Source: three-view drawing plus pictorial views. Frame: mm from the lowest corner of the part. Coordinates: 2 decimals unless noted, no trailing zeros. Write each loop counter-clockwise with the first axis right and the second up, starting at its lowest first coordinate (ties: lowest second). Pieces come first, ordered by that corner, then holes. Notation, with made-up numbers: M 8.5,31 L 32.5,31 A18 ccw 32.5,62 Z; hole C -20.5,69.25 d8. An arc over 180 degrees is marked long. Use CSV: the item, a comma, the result in double quotes.
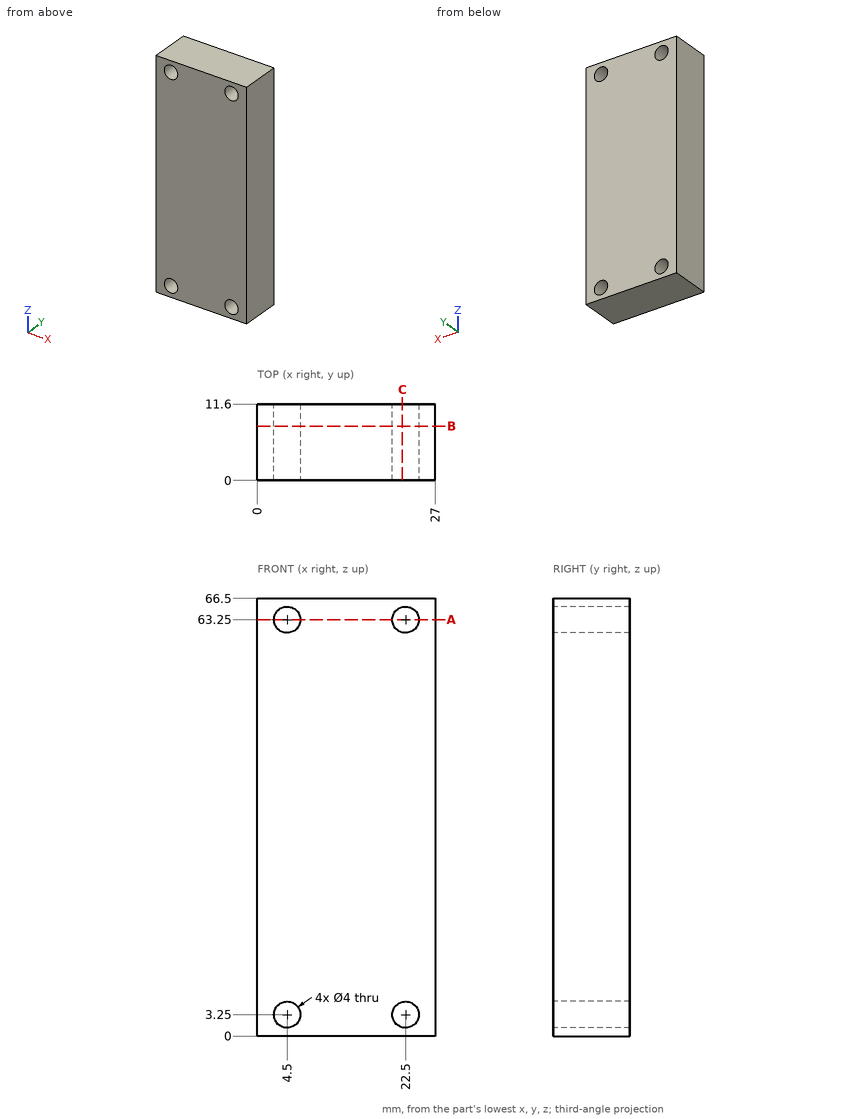
1. Material intervals for line 1 (Z direction, x = 4.5, y = 3.75); line 2 (Z direction, x = 5.25, y = 7.5), sorted ascending. Write a range as [from, to].
Resolved:
line 1,"z = [0, 1.25], [5.25, 61.25], [65.25, 66.5]"
line 2,"z = [0, 1.4], [5.1, 61.4], [65.1, 66.5]"
2. Section C-C (x = 22). Return loops of the section in (y, z), then the cut area to 3 significant figures.
Resolved:
outline,"M 0,0 L 11.6,0 L 11.6,1.31 L 0,1.31 Z; M 0,5.19 L 11.6,5.19 L 11.6,61.31 L 0,61.31 Z; M 0,65.19 L 11.6,65.19 L 11.6,66.5 L 0,66.5 Z"
area,"682 mm^2"
3. Section A-A (z = 63.25). Return loops of the section in (x, y), then the cut area to 3 significant figures.
Resolved:
outline,"M 0,0 L 2.5,0 L 2.5,11.6 L 0,11.6 Z; M 6.5,0 L 20.5,0 L 20.5,11.6 L 6.5,11.6 Z; M 24.5,0 L 27,0 L 27,11.6 L 24.5,11.6 Z"
area,"220 mm^2"
4. Section B-B (y = 8.25). Return loops of the section in (x, z), then the cut area to 3 significant figures.
Resolved:
outline,"M 0,0 L 27,0 L 27,66.5 L 0,66.5 Z; hole C 4.5,3.25 d4; hole C 4.5,63.25 d4; hole C 22.5,3.25 d4; hole C 22.5,63.25 d4"
area,"1,750 mm^2"
